Model file for the job. Use its own axes, mm. Round coordinates to 2 decimals unless told otherwise and drop trailing zeros. Loops run counter-clockwise (first coordinate to the right, second up) from the corner with the lowest first, then second, coordinate; pieces in that order, holes last. Notation, with made-up numbers: M -39.75,26.5 L -27.75,26.5 A30 cw -27.75,59.5 Z; hole C 67.5,78 d10. An arc over 180 degrees is marked long. Use a Markdown table: item, result. Add a question column.
Q1. Cut at B-B (z = -4). Give the cut face in (x, y) (1 decimal), plus the area to 3 significant figures.
Q2. Cut at D-D (y = 44.45). Give the cut face in (x, z) (1 decimal).
Q3. Probe line 1 (Z direction, x = -1.25, y = 182.5) (1 decimal); line 2 (Y direction, x = 0, z = 8.6). List the from-to ranges inside material, lowest first. Write a range as from..to.
Q4. Pin check, flat tips, straight feed: pin 1 (1.4 mm diameter, centred on y = 9.525, z = 0, fed in from -X); pin 2 (8 mm diameter, centred on x = 2, z = -3, fed in from +Y). Stop position of each tip, or through.
Q5. Cut at A-A (x = 0). Give the cut face in (y, z) (1 decimal), plus the area to 3 significant figures.
Q6. Cut at C-C (y = 443). Give the cut face in (x, z) (1 decimal), plus the area to 3 significant figures.
from build123d import *

# Parameters (mm, degrees)
SKETCH1_W           = 19.05
SKETCH1_H           = 19.05
SKETCH1_W_2         = 15.875
SKETCH1_H_2         = 15.875
BOSS_EXTRUDE1_DEPTH = 495.3
SKETCH2_R           = 4.9609375
CUT_EXTRUDE1_DEPTH  = 1.5875
CUT_EXTRUDE2_REACH  = 21.05
SKETCH3_R           = 0.889


with BuildPart() as part:
    # Sketch1 → Boss-Extrude1 (new body)
    with BuildSketch(Plane(origin=(0, 0, 0), x_dir=(1, 0, 0), z_dir=(0, 1, 0))):
        Rectangle(SKETCH1_W, SKETCH1_H)
        Rectangle(SKETCH1_W_2, SKETCH1_H_2, mode=Mode.SUBTRACT)
    extrude(amount=BOSS_EXTRUDE1_DEPTH)

    # Sketch2 → Cut-Extrude1 (cut)
    with BuildSketch(Plane.XY.offset(9.525)):
        with Locations((0, 44.45)):
            Circle(SKETCH2_R)
    extrude(amount=-CUT_EXTRUDE1_DEPTH, mode=Mode.SUBTRACT)

    # Sketch3 → Cut-Extrude2 (cut, up to next)
    with BuildSketch(Plane.ZY.offset(9.525), mode=Mode.PRIVATE) as cut_extrude2_sk1:
        with Locations((0, 9.525)):
            Circle(SKETCH3_R)
    cut_extrude2_tool1 = extrude(cut_extrude2_sk1.sketch, amount=-CUT_EXTRUDE2_REACH, mode=Mode.PRIVATE) & part.part
    add(cut_extrude2_tool1.solids().sort_by_distance((-9.525, 9.525, 0))[0], mode=Mode.SUBTRACT)


solid = part.part
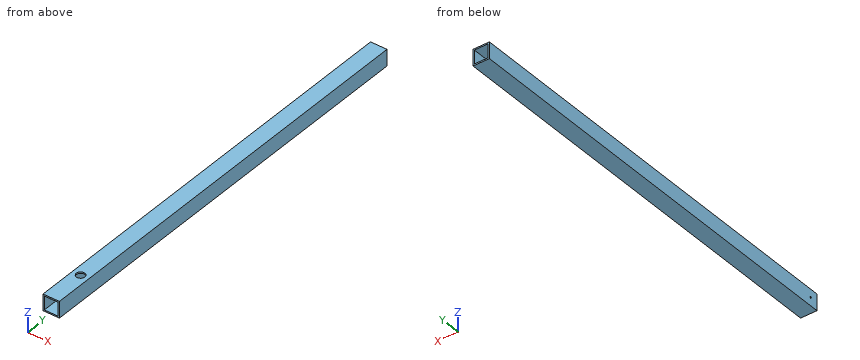
Checked values:
| question | item | result |
|---|---|---|
| 1 | outline | M -9.5,0 L -7.9,0 L -7.9,495.3 L -9.5,495.3 Z; M 7.9,0 L 9.5,0 L 9.5,495.3 L 7.9,495.3 Z |
| 1 | area | 1,570 mm^2 |
| 2 | outline | M -9.5,-9.5 L 9.5,-9.5 L 9.5,9.5 L 5,9.5 L 5,7.9 L 7.9,7.9 L 7.9,-7.9 L -7.9,-7.9 L -7.9,7.9 L -5,7.9 L -5,9.5 L -9.5,9.5 Z |
| 3 | line 1 | z = -9.5..-7.9, 7.9..9.5 |
| 3 | line 2 | y = 0..39.49, 49.41..495.3 |
| 4 | pin 1 | stops at x = 7.94 |
| 4 | pin 2 | passes through |
| 5 | outline | M 0,-9.5 L 495.3,-9.5 L 495.3,-7.9 L 0,-7.9 Z; M 0,7.9 L 39.5,7.9 L 39.5,9.5 L 0,9.5 Z; M 49.4,7.9 L 495.3,7.9 L 495.3,9.5 L 49.4,9.5 Z |
| 5 | area | 1,560 mm^2 |
| 6 | outline | M -9.5,-9.5 L 9.5,-9.5 L 9.5,9.5 L -9.5,9.5 Z; hole M -7.9,-7.9 L 7.9,-7.9 L 7.9,7.9 L -7.9,7.9 Z |
| 6 | area | 111 mm^2 |
